Check sheet for the drawn part. Datum: minimum x, y, z corner. Units: mm. A direction names the side the tool comes from. Coordinates: 2 decimals unless noted, no trailing zeros. Order: outer loops, then holes, each group sorted by start corner. A loop starts at its lowest first (then second) coordinate and runs counter-clockwise, first axis right, second up.
Q1. Cross-section at D-D, the plane z = 65.5. Record the boundary of the cut face in (x, y).
Q2. Cross-section at B-B, the plane y = 102. Record the boundary of the cut face in (x, z).
Q3. Cross-section at C-C, the plane x = 27.5. Record the boundary of the cut face in (y, z), and give its area (3 significant figures).
Q4. Set-up check for the marked faces 1 and 2: record each of +Z, -Z, +X, -X, +Y, -Y from which the full face is reachable in a straight line by a thin tool's end or side.
Q5. Thickness scan on line 1 (Y direction, x = 96.7, z = 40); line 2 (X direction, y = 28.5, z = 34.5); line 3 (Y direction, x = 73, z = 61). Record the ranges inside material, lowest first.
Q6. Depth check by flat-ended pin: P1, Ø4, axis at x = 96.5, z = 77, coming from the -Y side; P2, Ø5, axis at x = 40.5, z = 33.5, coming from the +Y side. Enter the tip coordinate at first touch or a pass-through.
Q7. Cross-section at A-A, the plane z = 40. Record the boundary of the cut face in (x, y), and give its area (3 significant figures).
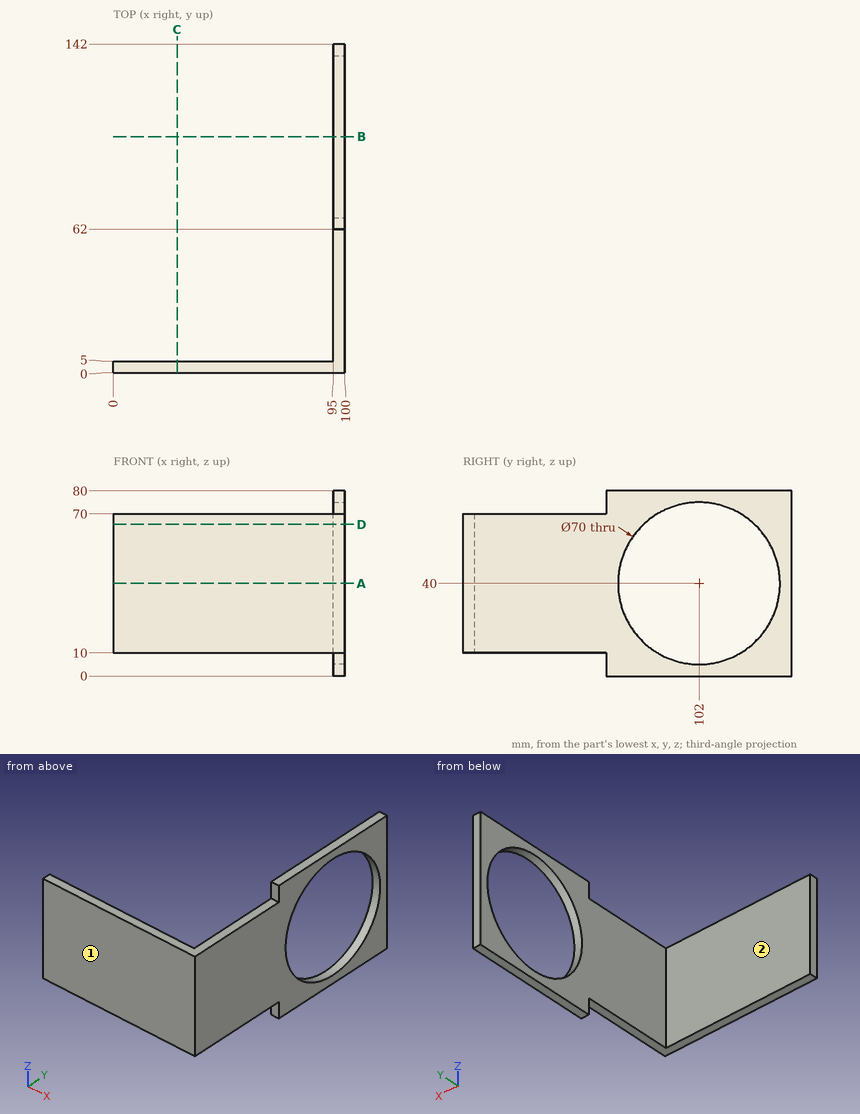
Check values:
1. outline: (0, 0) - (100, 0) - (100, 78.03) - (95, 78.03) - (95, 5) - (0, 5) - close; (95, 125.97) - (100, 125.97) - (100, 142) - (95, 142) - close
2. outline: (95, 0) - (100, 0) - (100, 5) - (95, 5) - close; (95, 75) - (100, 75) - (100, 80) - (95, 80) - close
3. outline: (0, 10) - (5, 10) - (5, 70) - (0, 70) - close
3. area: 300 mm2
4. face 1: +Z, -Z, +X, -X, -Y
4. face 2: +Z, -Z, -X, +Y
5. line 1: y = 0 to 67, 137 to 142
5. line 2: x = 95 to 100
5. line 3: y = 0 to 5
6. P1: stops at y = 62
6. P2: stops at y = 5
7. outline: (0, 0) - (100, 0) - (100, 67) - (95, 67) - (95, 5) - (0, 5) - close; (95, 137) - (100, 137) - (100, 142) - (95, 142) - close
7. area: 835 mm2
